from build123d import *

# Parameters (mm, degrees)
BOSS_EXTRUDE1_DEPTH = 6
SKETCH2_R           = 5.5179
CUT_EXTRUDE1_DEPTH  = 6.35
SKETCH4_R           = 2.5
BOSS_EXTRUDE2_DEPTH = 6.35


with BuildPart() as part:
    # Sketch1 → Boss-Extrude1 (new body)
    with BuildSketch(Plane(origin=(0, 0, 0), x_dir=(1, 0, 0), z_dir=(0, 1, 0))):
        with BuildLine():
            Line((0, 0), (70, 0))
            ThreePointArc((70, 0), (94.142135624, 10), (70, 20))
            Line((70, 20), (0, 20))
            Line((0, 20), (-16.12909928, 34.043913387))
            Line((-16.12909928, 34.043913387), (-40.507954262, 34.043913387))
            Line((-40.507954262, 34.043913387), (-40.507954262, 22.199626998))
            Line((-40.507954262, 22.199626998), (-9.850111043, 3.6873826))
            Line((-9.850111043, 3.6873826), (0, 0))
        make_face()
    extrude(amount=BOSS_EXTRUDE1_DEPTH)

    # Sketch2 → Cut-Extrude1 (cut)
    with BuildSketch(Plane(origin=(0, 6, 0), x_dir=(1, 0, 0), z_dir=(0, 1, 0))):
        with Locations((82.071067812, 10)):
            Circle(SKETCH2_R)
    extrude(amount=-CUT_EXTRUDE1_DEPTH, mode=Mode.SUBTRACT)

    # Sketch4 → Boss-Extrude2 (add)
    with BuildSketch(Plane(origin=(0, 0, 0), x_dir=(1, 0, 0), z_dir=(0, 1, 0))):
        with BuildLine():
            Line((-16.12909928, 34.043913387), (-23.200167092, 41.114981199))
            ThreePointArc((-23.200167092, 41.114981199), (-28.318526771, 43.235075195), (-33.436886451, 41.114981199))
            Line((-33.436886451, 41.114981199), (-40.507954262, 34.043913387))
            Line((-40.507954262, 34.043913387), (-16.12909928, 34.043913387))
        make_face()
        with Locations((-28.318526771, 39.615848358)):
            Circle(SKETCH4_R, mode=Mode.SUBTRACT)
    extrude(amount=BOSS_EXTRUDE2_DEPTH)


solid = part.part
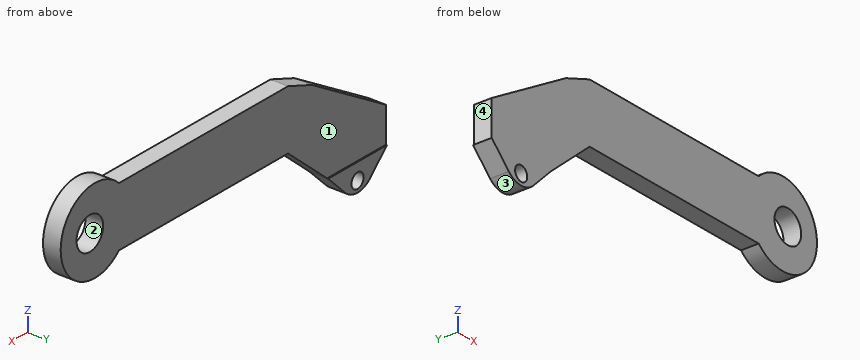
Read the model definition and answer for the solid it produces. Units are mm, in the model's axes. Face numbers are marked on the shaded views. Give positions to 0.01 mm unless a question says otherwise; leave off trailing zeros. Write each loop counter-clockwise with the first axis right and the second up, starting at its lowest first coordinate (ties: lowest second). Pieces come first, ordered by that corner, then holes. Notation, with made-up numbers: M -20,49 L -14,49 A31 ccw -14,76 Z; hole C -33,68.5 d5. An arc over 180 degrees is marked long. One line per item, written item: value. Start each with the question number.
(1) Find section B-B (x = 80). Determine the outline of the cut face in (y, z), plus the area to 3 significant figures.
(2) Flat-ended cylindrical pins translate along their axes: pin 1 Ø1 at (y, z) = (3, -35) entering from -X; pin 2 Ø3 at (x, y) = (42, 2.5) entering from -Z; pin 3 Ø1.8 at (x, y) = (25.5, 4) entering from +Z. Find the tip coordinate at first contact, or state that the pin passes through.
(3) Find the intervals of material crossed by line 1 (Y direction, x = 6.5, z = -12); line 2 (Z direction, x = 31.5, y = 3.5); line 3 (X direction, y = 4.25, z = -6), in increasing order.
(4) Find section A-A (z = -6). Determine the outline of the cut face in (x, y).
(5) Determine the mould class of the marked faces 1, 2, 3 and 4 for opening direction X: pulls with the +X half, pulls with the -X half, needs draft (parallel to the pull), parting line crosses it, or undercut.
(6) Find section D-D (x = 2.5). Determine the outline of the cut face in (y, z), plus the area to 3 significant figures.
(7) Find section C-C (y = 5). Determine the outline of the cut face in (x, z), plus the area to 3 significant figures.
Results below:
1. outline: M 0,-24.14 L 6,-24.14 L 6,-15.11 L 0,-15.11 Z; M 0,-4.89 L 6,-4.89 L 6,4.14 L 0,4.14 Z
1. area: 108 mm^2
2. pin 1: stops at x = -40.05
2. pin 2: stops at z = -20
2. pin 3: stops at z = 0
3. line 1: y = 0 to 6
3. line 2: z = -20 to 0
3. line 3: x = -13.68 to 78.27, 85.87 to 93.56
4. outline: M -13.68,0 L 78.27,0 L 78.27,6 L -13.68,6 Z; M 85.87,0 L 93.56,0 L 93.56,6 L 85.87,6 Z
5. face 1: needs draft
5. face 2: undercut
5. face 3: parting line crosses it
5. face 4: pulls with the -X half
6. outline: M 0,-20 L 6,-20 L 6,0 L 0,0 Z
6. area: 120 mm^2
7. outline: M -40.51,-34.04 L -33.44,-41.11 A7.24 ccw -23.2,-41.11 L -16.13,-34.04 L 0,-20 L 70,-20 A14.14 ccw long 70,0 L 0,0 L -9.85,-3.69 L -40.51,-22.2 Z; hole C -28.32,-39.62 d5; hole C 82.07,-10 d11.04
7. area: 2,840 mm^2
